```python
from build123d import *

# Parameters (mm, degrees)
BOSS_EXTRUDE1_DEPTH   = 4
F_4_0MM_DOWEL_HOLE1_D = 4


with BuildPart() as part:
    # Sketch1 → Boss-Extrude1 (new body)
    with BuildSketch(Plane(origin=(0, 0, 0), x_dir=(0, 0, -1), z_dir=(1, 0, 0))):
        Polygon((-46, 35), (-50, 35), (-50, 0), (0, 0), (0, 39), (-46, 39), align=None)
        Polygon((0, 39), (0, 0), (50, 0), (50, 35), (46, 35), (46, 39), align=None)
        Polygon((50, 0), (0, 0), (0, -39), (46, -39), (46, -35), (50, -35), align=None)
        Polygon((0, 0), (-50, 0), (-50, -35), (-46, -35), (-46, -39), (0, -39), align=None)
    extrude(amount=BOSS_EXTRUDE1_DEPTH)

    # Ø4.0mm Dowel Hole1 (through all)
    with Locations(Plane(origin=(0, -23.75, -39), x_dir=(0, 0, -1), z_dir=(-1, 0, 0))):
        with Locations((0, 0), (-78, -47.5)):
            Hole(F_4_0MM_DOWEL_HOLE1_D / 2)


solid = part.part
```
Geometry check sheet. Reference: the model listing, model coordinates, mm. A direction names the side the tool comes from. Give positions to 0.01 mm unless a question says otherwise; leave off trailing zeros. Write each loop counter-clockwise with the first axis right and the second up, starting at its lowest first coordinate (ties: lowest second). Pieces come first, ordered by that corner, then holes. Notation, with made-up numbers: (29.5, 67.25) -> (61.5, 67.25) arc R15 cw to (61.5, 75.25) -> close; hole circle Ø5 at (-30.75, -20). An arc over 180 degrees is marked (long way). One line per question, with ' | ' between items.
Item 1: Access from +Z, -Z, +X, -X, +Y, -Y to the whole of each face (thin tool, end or side, straight path). Record for faces 5 (the flat face through (2, -35, 48)), 6 (the flat face through (2, 37, 46)), 7 (the flat face through (2, 37, -46)), 8 (the flat face through (2, -37, -46)), 9 (the cylindrical face through (2.028, 22.398, 37.526)).
Determined:
face 5: +Z, +X, -X, -Y | face 6: +Z, +X, -X, +Y | face 7: -Z, +X, -X, +Y | face 8: -Z, +X, -X, -Y | face 9: +X, -X
Item 2: Sectioned sample at B-B, the plane y = -23.75. Record the boundary of the cut face in (x, z).
Determined:
outline: (0, -50) -> (4, -50) -> (4, -41) -> (0, -41) -> close; (0, -37) -> (4, -37) -> (4, 50) -> (0, 50) -> close
Item 3: Scan lines: line 1 along Y through (x, z) = (2.3, -39); line 2 along Y through (x, z) = (1.15, 39); line 3 along Z through (x, y) = (2.15, -23.75). Record each from-to range of solid material in increasing order.
Determined:
line 1: -39 to -25.75, -21.75 to 39 | line 2: -39 to 21.75, 25.75 to 39 | line 3: -50 to -41, -37 to 50
Item 4: Depth check by flat-ended pin: pin 1 (3.5 mm diameter, centred on y = 23.75, z = 39, fed in from +X); pin 2 (2 mm diameter, centred on x = 1.5, y = -36.5, fed in from +Z); pin 3 (2 mm diameter, centred on x = 2.5, z = -48.5, fed in from -Y); pin 4 (2 mm diameter, centred on x = 1.5, z = -49, fed in from +Y). Enter the tip coordinate at first touch or a pass-through.
Determined:
pin 1: through | pin 2: z = 46 | pin 3: y = -35 | pin 4: y = 35
Item 5: Sectioned sample at A-A, the plane z = 39. Record the boundary of the cut face in (x, y).
Determined:
outline: (0, -39) -> (4, -39) -> (4, 21.75) -> (0, 21.75) -> close; (0, 25.75) -> (4, 25.75) -> (4, 39) -> (0, 39) -> close
Item 6: Draft check along Z on faces 1 (the flat face through (2, -35, -48)), 2 (the flat face through (2, 0, -50)), 3 (the cylindrical face through (2.028, -22.533, -40.587)), 4 (the flat face through (2, -37, 46)). Enter one of: released by +Z, released by -Z, zero draft, split by the parting line, or undercut.
Determined:
face 1: zero draft | face 2: released by -Z | face 3: undercut | face 4: released by +Z
